Part print with two shaded views. Sizes in mm from the minimum x, y, z corner. A direction names the side the tool comes from. Round coordinates to 2 decimals unless told otherwise and drop trailing zeros. Write each loop counter-clockwise with the first axis right and the second up, starting at its lowest first coordinate (ties: lowest second). Pieces come first, ordered by that corner, then holes. Notation, with made-up numbers: (29.25, 89) -> (75.25, 89) arc R24 cw to (75.25, 107) -> close; hole circle Ø8 at (-29, 8). An arc over 180 degrees is marked (long way). Answer as CSV lines item,"result".
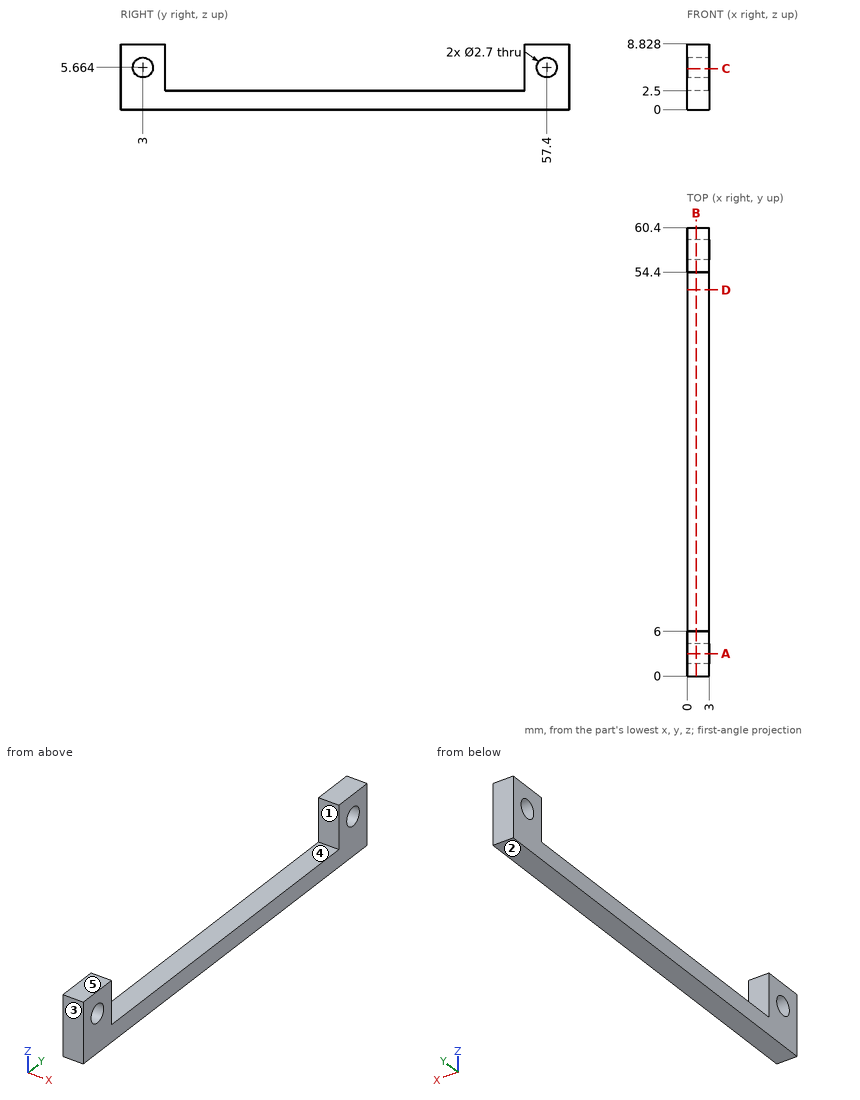
1. Cut at C-C, the plane z = 5.5. Write the cut outline in (x, y).
Results found:
outline,"(0, 0) -> (3, 0) -> (3, 1.66) -> (0, 1.66) -> close; (0, 4.34) -> (3, 4.34) -> (3, 6) -> (0, 6) -> close; (0, 54.4) -> (3, 54.4) -> (3, 56.06) -> (0, 56.06) -> close; (0, 58.74) -> (3, 58.74) -> (3, 60.4) -> (0, 60.4) -> close"
2. Which spindle directions (+Z, -Z, +X, -X, +Y, -Y) get a long thin tool onto all of the face, cutting with end or side? Do the marked faces 4 and 5. Say none if no direction does.
Results found:
face 4,"+Z, +X, -X"
face 5,"+Z, +X, -X, +Y, -Y"
3. Probe line 1 along Y through (x, z) = (1.8, 5.5); line 2 along Y through (x, z) = (1.9, 8.25); line 3 along Z through (x, y) = (1.05, 27.5). List the from-to ranges inside material, lowest first.
Results found:
line 1,"y = 0 to 1.66, 4.34 to 6, 54.4 to 56.06, 58.74 to 60.4"
line 2,"y = 0 to 6, 54.4 to 60.4"
line 3,"z = 0 to 2.5"
4. Cut at D-D, the plane y = 52. Write the cut outline in (x, z).
Results found:
outline,"(0, 0) -> (3, 0) -> (3, 2.5) -> (0, 2.5) -> close"
5. Cut at A-A, the plane y = 3. Write the cut outline in (x, z).
Results found:
outline,"(0, 0) -> (3, 0) -> (3, 4.31) -> (0, 4.31) -> close; (0, 7.01) -> (3, 7.01) -> (3, 8.83) -> (0, 8.83) -> close"
6. Mould opens along Y. For the marked faces 1, 2 and 3 say: +Y half, -Y half, draft (parallel to the pull), parting line (faces both ways), or undercut.
Results found:
face 1,"undercut"
face 2,"draft"
face 3,"-Y half"
7. Cut at B-B, the plane x = 1.2. Write the cut outline in (y, z).
Results found:
outline,"(0, 0) -> (60.4, 0) -> (60.4, 8.83) -> (54.4, 8.83) -> (54.4, 2.5) -> (6, 2.5) -> (6, 8.83) -> (0, 8.83) -> close; hole circle Ø2.7 at (3, 5.66); hole circle Ø2.7 at (57.4, 5.66)"
8. Drop a flat-ended pin along its axis: pin 1 Ø1.5 at (x, y) = (1.5, 52) entering from +Z. Give the stop position or say it passes through.
Results found:
pin 1,"stops at z = 2.5"
